```python
from build123d import *

# Parameters (mm, degrees)
RESSALTO_EXTRUS_O1_DEPTH = 1
ESBO_O2_W                = 5
ESBO_O2_H                = 5
RESSALTO_EXTRUS_O2_DEPTH = 6


with BuildPart() as part:
    # Esboço1 → Ressalto-extrusão1 (new body)
    with BuildSketch(Plane(origin=(0, 0, 0), x_dir=(1, 0, 0), z_dir=(0, 1, 0))):
        Polygon((-21.795929641, 4.783320054), (-12.808127222, -4.204482365), (-12.808127222, 35.123446913), (-6.91286311, 41.018711025), (-2.185714729, 41.018711025), (5.111319205, 48.315744958), (10.733649893, 48.315744958), (13.872231707, 45.177163144), (21.962429244, 45.177163144), (26.174966365, 40.964626022), (26.174966365, 38.275642193), (27.35031576, 37.100292798), (33.357124102, 37.100292798), (37.825539643, 32.631877257), (37.825539643, -32.506234834), (22.369869311, -47.961905165), (-2.211409105, -47.961905165), (-37.585857198, -12.587457072), (-37.585857198, 0.447182703), (-33.249719847, 4.783320054), align=None)
    extrude(amount=RESSALTO_EXTRUS_O1_DEPTH)

    # Esboço2 → Ressalto-extrusão2 (add)
    with BuildSketch(Plane(origin=(0, 1, 0), x_dir=(1, 0, 0), z_dir=(0, 1, 0))):
        with Locations((29.396408855, 29.306282823)):
            Rectangle(ESBO_O2_W, ESBO_O2_H)
        with Locations((-7.255035982, 29.306282823)):
            Rectangle(ESBO_O2_W, ESBO_O2_H)
    extrude(amount=RESSALTO_EXTRUS_O2_DEPTH)


solid = part.part
```
Here's how the part is built. I have some questions about the finished solid (model axes, mm). A direction names the side the tool comes from. Coordinates: 2 decimals unless noted, no trailing zeros. Order: outer loops, then holes, each group sorted by start corner. A loop starts at its lowest first (then second) coordinate and runs counter-clockwise, first axis right, second up. Notation, with made-up numbers: M -31.5,49.5 L -17.5,49.5 A22 ccw -17.5,57.5 Z; hole C 89.25,-28.5 d2. An arc over 180 degrees is marked long. Answer as a JSON object with one key per item and string values. Group by question number.
(1) If we mould it in two halves opening along X, with no side actions, what happens to faces 6 (the face through (-7, 4, -31.806)), 7 (the face through (-17.36, 0.49, -0.35)), 8 (the face through (-35.448, 0.493, -2.585)), 9 (the face through (24.04, 0.49, -43.1))? For each: released by +X, released by -X, zero draft, split by the parting line, or undercut.
(2) For pin 1 (1.5 mm diameter, centred on x = 30, y = 3.5, fed in from +Z); pin 2 (2.5 mm diameter, centred on y = 4, z = -30, fed in from +X); pin 3 (0.8 mm diameter, centred on x = 17, y = 0.5, fed in from -Z), each with a flat end and sliding along its axis, tell me the tip position at first contact or that it passes through.
(3) Suppose I cut it at B-B, the plane z = -9. Please give me the cut outline in (x, y).
(4) Suppose I cut it at C-C, the plane x = -19. Please give me the cut outline in (y, z).
(5) I need wall thicknesses on probe 1 along Z at (x, y) = (28.5, 4.25); probe 2 along Y at (x, z) = (-20, 0). Which ranges of each line are inside material? Lowest first, please.
(6) Which directions (+Z, -Z, +X, -X, +Y, -Y) give clear straight access to the entire face, cutting with the end or side of a thin tool? Please do faces 1 (the face through (29, 4, -26.806)), 2 (the face through (30.206, 0.493, 40.126)), 3 (the face through (26.896, 4, -29)), 4 (the face through (-19.651, 0.493, 30.522)), 5 (the face through (31.896, 4, -29)).
(7) Suppose I cut it at A-A, the plane y = 3.5. Please give me the cut outline in (x, z), then the cut area to 3 significant figures.
Values found:
{
 "1": {"face 6": "zero draft", "face 7": "undercut", "face 8": "released by -X", "face 9": "released by +X"},
 "2": {"pin 1": "stops at z = -26.81", "pin 2": "stops at x = 31.9", "pin 3": "stops at z = -45.18"},
 "3": {"outline": "M -12.81,0 L 37.83,0 L 37.83,1 L -12.81,1 Z"},
 "4": {"outline": "M 0,-1.99 L 1,-1.99 L 1,31.17 L 0,31.17 Z"},
 "5": {"probe 1": "z = -31.81 to -26.81", "probe 2": "y = 0 to 1"},
 "6": {"face 1": "+Z, +X, -X, +Y", "face 2": "+Z, +X, +Y, -Y", "face 3": "+Z, -Z, +Y", "face 4": "+Z, -X, +Y, -Y", "face 5": "+Z, -Z, +X, +Y"},
 "7": {"outline": "M -9.76,-31.81 L -4.76,-31.81 L -4.76,-26.81 L -9.76,-26.81 Z; M 26.9,-31.81 L 31.9,-31.81 L 31.9,-26.81 L 26.9,-26.81 Z", "area": "50.0 mm^2"}
}
